```python
from build123d import *

# Parameters (mm, degrees)
F0_W     = 21.5
F0_H     = 21.4
F1_DEPTH = 1
F0_H_2   = 4
F2_DEPTH = 3
F4_D     = 2.85
F5_R     = 2


# Not quite as in the source:
# - a feature names something its author has since deleted; it is built from what else it names


with BuildPart() as f1:
    # F0 (on Top) → F1 (new body)
    with BuildSketch(Plane.XY):
        Rectangle(F0_W, F0_H)
    extrude(amount=F1_DEPTH)

    # F0 (on Top) → F2 (join)
    with BuildSketch(Plane.XY):
        with Locations((0, 12.7)):
            Rectangle(F0_W, F0_H_2)
    extrude(amount=F2_DEPTH)

    # F4 (through all)
    with Locations(Plane.YZ.offset(10.75)):
        with Locations((12.7, 2)):
            Hole(F4_D / 2)

    # F5
    f5_edges = [f1.edges().sort_by_distance(p)[0] for p in [
        (0, 14.7, 0),
    ]]
    fillet(f5_edges, radius=F5_R)


solid = f1.part
```
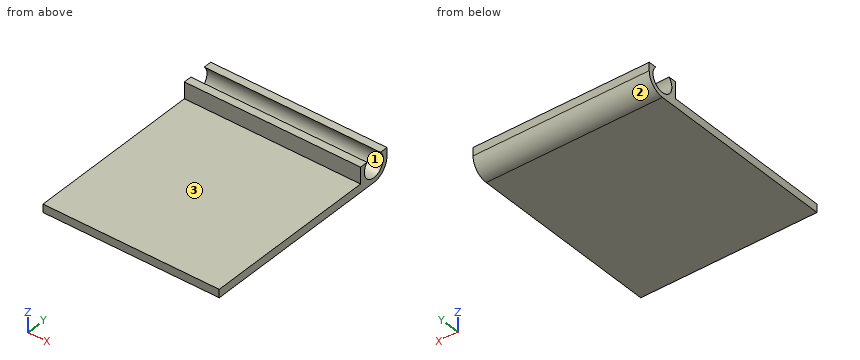
The listing builds one solid part. Answer for the finished solid, in the listing's coordinates (mm). Face numbers are marked on the shaded views. Give positions to 0.01 mm unless a question says otherwise; leave off trailing zeros. Write each loop counter-clockwise with the first axis right and the second up, starting at its lowest first coordinate (ties: lowest second). Pieces come first, ordered by that corner, then holes. Notation, with made-up numbers: (13, 56.25) - (45, 56.25) arc R12 cw to (45, 63.25) - close; hole circle Ø9 at (-39, 14.25). An arc over 180 degrees is marked (long way). Use one line per item in the form item = value. Start each with the question number.
1) Find section C-C on y = -2.75. Determine the outline of the cut face in (x, z).
2) Find section B-B on z = 2.4. Determine the outline of the cut face in (x, y), plus the area to 3 significant figures.
3) Flat-ended cylindrical pins translate along their axes: pin 1 Ø1 at (x, y) = (7, 3) entering from +Z; pin 2 Ø1 at (x, z) = (4.5, 2) entering from -Y. Find the tip coordinate at first contact, or state that the pin passes through.
4) Find section A-A on x = 8.25. Determine the outline of the cut face in (y, z) (3 decimals), plus the area to 3 significant figures.
5) The mould has two halves that part along Y. Classify the marked faces 1, 2 and 3: pulls with the +Y half, pulls with the -Y half, needs draft (parallel to the pull), parting line crosses it, or undercut.
6) Consider line 1 along Y through (x, z) = (5.25, 2) (3 decimals); line 2 along Z through (x, y) = (1.5, 4.25); line 3 along Z through (x, y) = (3.5, 12.7) (3 decimals). Determine where each line is inside the solid, lowest interval first. Write a range as from..to.
7) Find section D-D on z = 0.3. Determine the outline of the cut face in (x, y).
Geometry results:
q1.outline = (-10.75, 0) - (10.75, 0) - (10.75, 1) - (-10.75, 1) - close
q2.outline = (-10.75, 10.7) - (10.75, 10.7) - (10.75, 11.33) - (-10.75, 11.33) - close; (-10.75, 14.07) - (10.75, 14.07) - (10.75, 14.7) - (-10.75, 14.7) - close
q2.area = 27.2 mm2
q3.pin_1 = 1
q3.pin_2 = 10.7
q4.outline = (-10.7, 0) - (12.7, 0) arc R2 ccw to (14.7, 2) - (14.7, 3) - (13.715, 3) arc R1.425 cw (long way) to (11.685, 3) - (10.7, 3) - (10.7, 1) - (-10.7, 1) - close
q4.area = 26.8 mm2
q5.face_1 = undercut
q5.face_2 = pulls with the +Y half
q5.face_3 = needs draft
q6.line_1 = 10.7..11.275, 14.125..14.7
q6.line_2 = 0..1
q6.line_3 = 0..0.575
q7.outline = (-10.75, -10.7) - (10.75, -10.7) - (10.75, 13.75) - (-10.75, 13.75) - close
